from build123d import *

# Parameters (mm, degrees)
F0_W     = 106
F0_H     = 58
F1_DEPTH = 52
F2_W     = 62
F2_H     = 26
F3_DEPTH = 52.001
F4_W     = 36
F4_H     = 27
F5_DEPTH = 90
F7_DEPTH = 18


with BuildPart() as f1:
    # F0 (on Front) → F1 (new body)
    with BuildSketch(Plane.XZ):
        with Locations((53, 29)):
            Rectangle(F0_W, F0_H)
    extrude(amount=F1_DEPTH)

    # F2 (on face) → F3 (cut, through all)
    with BuildSketch(Plane.XZ.offset(52)):
        with Locations((31, 45)):
            Rectangle(F2_W, F2_H)
    extrude(amount=-F3_DEPTH, mode=Mode.SUBTRACT)

    # F4 (on face) → F5 (cut)
    with BuildSketch(Plane.YZ.offset(106)):
        with Locations((-18, 31.5)):
            Rectangle(F4_W, F4_H)
    extrude(amount=-F5_DEPTH, mode=Mode.SUBTRACT)

    # F6 (on face) → F7 (cut)
    with BuildSketch(Plane(origin=(0, 0, 0), x_dir=(1, 0, 0), z_dir=(0, 0, -1))):
        with BuildLine():
            ThreePointArc((82, 27), (76.343146, 13.343146), (90, 19))
            Line((90, 19), (82, 19))
            Line((82, 19), (82, 27))
        make_face()
        with BuildLine():
            Line((82, 19), (90, 19))
            ThreePointArc((90, 19), (87.656854, 24.656854), (82, 27))
            Line((82, 27), (82, 19))
        make_face()
        with BuildLine():
            ThreePointArc((45, 19), (42.656854, 24.656854), (37, 27))
            ThreePointArc((37, 27), (31.343146, 13.343146), (45, 19))
        make_face()
    extrude(amount=-F7_DEPTH, mode=Mode.SUBTRACT)


solid = f1.part
The model under review builds one solid part; all positions refer to its coordinate system, in mm. A direction names the side the tool comes from. Round coordinates to 2 decimals unless told otherwise and drop trailing zeros. Write each loop counter-clockwise with the first axis right and the second up, starting at its lowest first coordinate (ties: lowest second). Pieces come first, ordered by that corner, then holes. Notation, with made-up numbers: M 12,46 L 27,46 A30 ccw 27,82 Z; hole C 71,-4.75 d9. An arc over 180 degrees is marked long. Use a Markdown table: item, result. Add a question column.
Q1. Insertion check: pin 1 (21.5 mm diameter, centred on x = 70.5, z = 36, fed in from +Y); pin 2 (13 mm diameter, centred on x = 82, y = -19, fed in from -Z). Each pin has a flat end and moves straight along its axis. Give the tip position at first contact, or say it passes through.
Q2. We need section D-D, the plane x = 47. State the section outline as (y, z) points.
Q3. We need section B-B, the plane x = 87.5. State the section outline as (y, z) points.
Q4. The part is to be moulded in two halves that separate along Z. For faces 1 (the face through (16, -18, 25)), 2 (the face through (84, -26, 58)), 3 (the face through (62, -18, 18)), say which applies: pulls with the +Z half, pulls with the -Z half, needs draft (parallel to the pull), parting line crosses it, or undercut.
Q5. We need section C-C, the plane z = 29. State the section outline as (x, y) points.
Q6. To check wall thickness, follow line 1 (X direction, y = -19, z = 6); line 2 (Z direction, x = 65.5, y = -31); line 3 (Y direction, x = 82, z = 13.75). State the ranges of each line that lie inside material, in increasing order.
Q7. Machinability: for faces 4 (the face through (24, -38, 32)), 5 (the face through (72, -36, 28)), 6 (the face through (84, -18, 45)), which of the approach directions +Z, -Z, +X, -X, +Y, -Y give a long, thin tool a straight path to every point of the face, cutting with its end or side? Answer none if there is none.
Q8. We need section A-A, the plane z = 14.5. State the section outline as (x, y) points.
Findings below:
| question | item | result |
|---|---|---|
| 1 | pin 1 | stops at y = 0 |
| 1 | pin 2 | stops at z = 45 |
| 2 | outline | M -52,0 L 0,0 L 0,18 L -36,18 L -36,32 L -52,32 Z |
| 3 | outline | M -52,0 L -24.81,0 L -24.81,18 L -36,18 L -36,45 L 0,45 L 0,58 L -52,58 Z; M -13.19,0 L 0,0 L 0,18 L -13.19,18 Z |
| 4 | face 1 | needs draft |
| 4 | face 2 | pulls with the +Z half |
| 4 | face 3 | undercut |
| 5 | outline | M 0,-52 L 106,-52 L 106,-36 L 16,-36 L 16,0 L 0,0 Z |
| 6 | line 1 | x = 0 to 29, 45 to 74, 90 to 106 |
| 6 | line 2 | z = 0 to 18, 45 to 58 |
| 6 | line 3 | y = -52 to -27, -11 to 0 |
| 7 | face 4 | +Z, -X, +Y, -Y |
| 7 | face 5 | +X, +Y |
| 7 | face 6 | +X, -X, +Y |
| 8 | outline | M 0,-52 L 106,-52 L 106,0 L 0,0 Z; hole C 37,-19 d16; hole C 82,-19 d16 |
